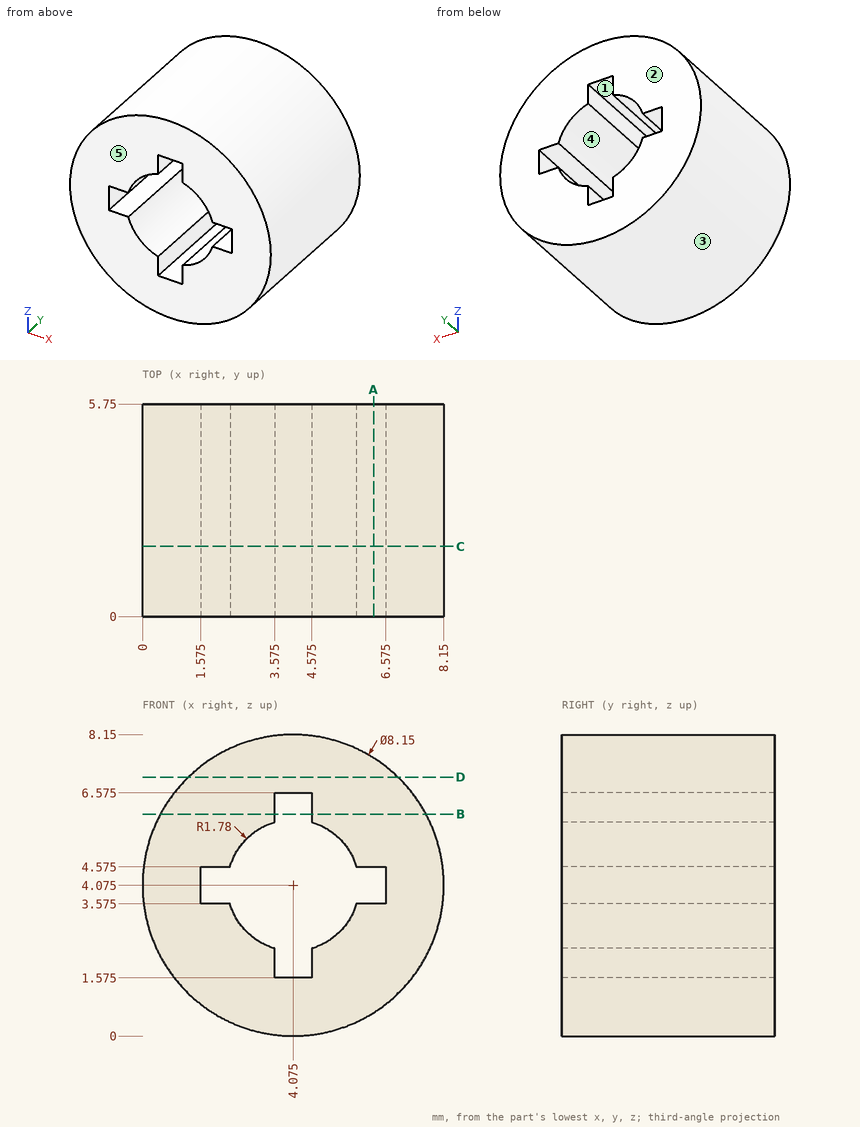
Input: dimensioned drawing with shaded views. Units: mm. Origin: part minimum x, y, z. A direction names the side the tool comes from. Coordinates: 2 decimals unless noted, no trailing zeros. Order: outer loops, then holes, each group sorted by start corner. A loop starts at its lowest first (then second) coordinate and runs counter-clockwise, first axis right, second up.
(1) Section query B-B (z = 6). Return the cut outline in (x, y) (3 decimals).
(2) Section query D-D (z = 7). Return the cut outline in (x, y), plus the area to 3 significant figures.
(3) Draft query along X for the marked faces 3, 4 and 5. Return one class per face: pulls with the +X half, pulls with the -X half, needs draft (parallel to the pull), parting line crosses it, or undercut.
(4) Section query A-A (x = 6.25). Return the cut outline in (y, z) (3 decimals), plus the area to 3 significant figures.
(5) Access query for the marked faces 1 and 2. Directions: +Z, -Z, +X, -X, +Y, -Y. A direction counts if a zero-diameter tool reaches every point of the face in a straight line with its end or side. Return the directions, or none.
(6) First-contact query: pin 1 (0.6 mm diameter, centred on y = 3.5, z = 2, fed in from +X); pin 2 (0.9 mm diameter, centred on x = 2, y = 2, fed in from +Z); pin 3 (1.5 mm diameter, centred on x = 2.5, y = 2.5, fed in from -Z). Flat tips, straight axial feed; report the tip coordinate or a pass-through.
(7) Material intervals for probe 1 along Z at (x, y) = (6.5, 1.25) (3 decimals); probe 2 along X at (y, z) = (2.65, 6.25) (3 decimals); probe 3 along X at (y, z) = (1.95, 3.25), sorted ascending.
(8) Section query C-C (y = 1.9). Return the cut outline in (x, z) (3 decimals).
Solution:
1. outline: (0.483, 0) - (3.575, 0) - (3.575, 5.75) - (0.483, 5.75) - close; (4.575, 0) - (7.667, 0) - (7.667, 5.75) - (4.575, 5.75) - close
2. outline: (1.24, 0) - (6.91, 0) - (6.91, 5.75) - (1.24, 5.75) - close
2. area: 32.6 mm2
3. face 3: parting line crosses it
3. face 4: undercut
3. face 5: needs draft
4. outline: (0, 0.629) - (5.75, 0.629) - (5.75, 3.575) - (0, 3.575) - close; (0, 4.575) - (5.75, 4.575) - (5.75, 7.521) - (0, 7.521) - close
4. area: 33.9 mm2
5. face 1: +Y, -Y
5. face 2: +Z, -Z, +X, -X, +Y
6. pin 1: stops at x = 7.74
6. pin 2: stops at z = 7.81
6. pin 3: stops at z = 0.08
7. probe 1: z = 0.8 to 3.575, 4.575 to 7.35
7. probe 2: x = 0.629 to 3.575, 4.575 to 7.521
7. probe 3: x = 0.08 to 2.5, 5.65 to 8.07
8. outline: circle Ø8.15 at (4.075, 4.075); hole (1.575, 3.575) - (2.367, 3.575) arc R1.78 ccw to (3.575, 2.367) - (3.575, 1.575) - (4.575, 1.575) - (4.575, 2.367) arc R1.78 ccw to (5.783, 3.575) - (6.575, 3.575) - (6.575, 4.575) - (5.783, 4.575) arc R1.78 ccw to (4.575, 5.783) - (4.575, 6.575) - (3.575, 6.575) - (3.575, 5.783) arc R1.78 ccw to (2.367, 4.575) - (1.575, 4.575) - close
